Input: part model. Units: mm. Frame: model coordinates. A direction names the side the tool comes from. Give positions to 0.01 mm unless a question says otherwise; leave off trailing zeros. Loops run counter-clockwise (first coordinate to the right, second up) from the corner with the lowest first, then second, coordinate; pieces in that order, holes last. Notation, with made-up numbers: (72, 51) -> (78, 51) arc R24 cw to (78, 88) -> close; hole circle Ø11 at (29, 16.5). An arc over 180 degrees is marked (long way). One line per question, with ' | ' between items.
from build123d import *

# Parameters (mm, degrees)
SKETCH_1_R          = 1.45
EXTRUDE_1_DEPTH     = 1
SKETCH_2_W          = 3.674905937
SKETCH_2_H          = 8.103638732
EXTRUDE_2_DEPTH     = 4.6
SKETCH_3_W          = 9.2
SKETCH_3_H          = 9.2
EXTRUDE_3_DEPTH     = 3
SKETCH_4_R          = 3.75
EXTRUDE_4_DEPTH     = 3.8
SKETCH_5_W          = 5.32390219
SKETCH_5_H          = 6.666656283
EXTRUDE_5_DEPTH     = 2.2
SKETCH_6_W          = 12.46284852
SKETCH_6_H          = 12.975244807
EXTRUDE_6_DEPTH     = 1.7
SKETCH_7_W          = 10.69456342
SKETCH_7_H          = 13.354174441
EXTRUDE_7_DEPTH     = 1
SKETCH_8_W          = 14.555394544
SKETCH_8_H          = 14.555394544
EXTRUDE_8_DEPTH     = 6
SKETCH_9_W          = 18.172258066
SKETCH_9_H          = 5.460745639
EXTRUDE_9_DEPTH     = 2.5
SKETCH_10_W         = 17.57536677
SKETCH_10_H         = 2.2
CUT_EXTRUDE_1_DEPTH = 4.5


with BuildPart() as part:
    # 草图1 → 凸台-拉伸1 (new body)
    with BuildSketch(Plane(origin=(0, 0, 0), x_dir=(1, 0, 0), z_dir=(0, 1, 0))):
        with BuildLine():
            Line((-11, 17.5), (11, 17.5))
            ThreePointArc((11, 17.5), (11.707106781, 17.207106781), (12, 16.5))
            Line((12, 16.5), (12, 12.3))
            ThreePointArc((12, 12.3), (12.527207794, 11.027207794), (13.8, 10.5))
            Line((13.8, 10.5), (18, 10.5))
            ThreePointArc((18, 10.5), (18.707106781, 10.207106781), (19, 9.5))
            Line((19, 9.5), (19, -9.5))
            ThreePointArc((19, -9.5), (18.707106781, -10.207106781), (18, -10.5))
            Line((18, -10.5), (13.8, -10.5))
            ThreePointArc((13.8, -10.5), (12.527207794, -11.027207794), (12, -12.3))
            Line((12, -12.3), (12, -16.5))
            ThreePointArc((12, -16.5), (11.707106781, -17.207106781), (11, -17.5))
            Line((11, -17.5), (-11, -17.5))
            ThreePointArc((-11, -17.5), (-11.707106781, -17.207106781), (-12, -16.5))
            Line((-12, -16.5), (-12, -12.3))
            ThreePointArc((-12, -12.3), (-12.527207794, -11.027207794), (-13.8, -10.5))
            Line((-13.8, -10.5), (-18, -10.5))
            ThreePointArc((-18, -10.5), (-18.707106781, -10.207106781), (-19, -9.5))
            Line((-19, -9.5), (-19, 9.5))
            ThreePointArc((-19, 9.5), (-18.707106781, 10.207106781), (-18, 10.5))
            Line((-18, 10.5), (-13.8, 10.5))
            ThreePointArc((-13.8, 10.5), (-12.527207794, 11.027207794), (-12, 12.3))
            Line((-12, 12.3), (-12, 16.5))
            ThreePointArc((-12, 16.5), (-11.707106781, 17.207106781), (-11, 17.5))
        make_face()
        with Locations((15.875, 7.375)):
            Circle(SKETCH_1_R, mode=Mode.SUBTRACT)
        with Locations((15.875, -7.375)):
            Circle(SKETCH_1_R, mode=Mode.SUBTRACT)
        with Locations((-15.875, -7.375)):
            Circle(SKETCH_1_R, mode=Mode.SUBTRACT)
        with Locations((-15.875, 7.375)):
            Circle(SKETCH_1_R, mode=Mode.SUBTRACT)
    extrude(amount=EXTRUDE_1_DEPTH)

    # 草图2 → 凸台-拉伸2 (add)
    with BuildSketch(Plane(origin=(0, 1, 0), x_dir=(1, 0, 0), z_dir=(0, 1, 0))):
        with Locations((-17.008218503, 0.494698876)):
            Rectangle(SKETCH_2_W, SKETCH_2_H)
    extrude(amount=EXTRUDE_2_DEPTH)

    # 草图3 → 凸台-拉伸3 (add)
    with BuildSketch(Plane(origin=(0, 1, 0), x_dir=(1, 0, 0), z_dir=(0, 1, 0))):
        with Locations((0, 9.9)):
            Rectangle(SKETCH_3_W, SKETCH_3_H)
    extrude(amount=EXTRUDE_3_DEPTH)

    # 草图4 → 凸台-拉伸4 (add)
    with BuildSketch(Plane(origin=(0, 4, 0), x_dir=(1, 0, 0), z_dir=(0, 1, 0))):
        with Locations((0, 10.082434237)):
            Circle(SKETCH_4_R)
    extrude(amount=EXTRUDE_4_DEPTH)

    # 草图5 → 凸台-拉伸5 (add)
    with BuildSketch(Plane(origin=(0, 1, 0), x_dir=(1, 0, 0), z_dir=(0, 1, 0))):
        with Locations((16.560633805, 0.129563992)):
            Rectangle(SKETCH_5_W, SKETCH_5_H)
    extrude(amount=EXTRUDE_5_DEPTH)

    # 草图6 → 凸台-拉伸6 (add)
    with BuildSketch(Plane(origin=(0, 1, 0), x_dir=(1, 0, 0), z_dir=(0, 1, 0))):
        with Locations((0, -10.346273638)):
            Rectangle(SKETCH_6_W, SKETCH_6_H)
    extrude(amount=EXTRUDE_6_DEPTH)

    # 草图7 → 凸台-拉伸7 (add)
    with BuildSketch(Plane(origin=(0, 1, 0), x_dir=(1, 0, 0), z_dir=(0, 1, 0))):
        with Locations((0, -13.384558474)):
            Rectangle(SKETCH_7_W, SKETCH_7_H)
    extrude(amount=EXTRUDE_7_DEPTH)

    # 草图8 → 凸台-拉伸8 (add)
    with BuildSketch(Plane.XZ):
        Rectangle(SKETCH_8_W, SKETCH_8_H)
    extrude(amount=EXTRUDE_8_DEPTH)

    # 草图9 → 凸台-拉伸9 (add)
    with BuildSketch(Plane.XZ):
        with Locations((0, -13.73622766)):
            Rectangle(SKETCH_9_W, SKETCH_9_H)
    extrude(amount=EXTRUDE_9_DEPTH)

    # 草图10 → 切除-拉伸1 (cut)
    with BuildSketch(Plane.XZ.offset(6)):
        with Locations((-0.008749504, 5.958042987)):
            Rectangle(SKETCH_10_W, SKETCH_10_H)
        with Locations((-0.008749504, 2.958042987)):
            Rectangle(SKETCH_10_W, SKETCH_10_H)
        with Locations((-0.008749504, -0.041957013)):
            Rectangle(SKETCH_10_W, SKETCH_10_H)
        with Locations((-0.008749504, -3.041957013)):
            Rectangle(SKETCH_10_W, SKETCH_10_H)
        with Locations((-0.008749504, -6.041957013)):
            Rectangle(SKETCH_10_W, SKETCH_10_H)
    extrude(amount=-CUT_EXTRUDE_1_DEPTH, mode=Mode.SUBTRACT)


solid = part.part
1. Pin query (flat end, axial travel): P1, Ø4, axis at y = -3, z = 1.5, coming from the +X side; P2, Ø2.5, axis at y = 3, z = -10.5, coming from the +X side; P3, Ø1.7, axis at x = 15.875, z = 7.375, coming from the +Y side; P4, Ø1.8, axis at x = 3.5, y = -4, coming from the -Z side. Return the tip coordinate at first contact, or that it passes through.
Determined:
P1: stops at x = 7.28 | P2: stops at x = 4.6 | P3: passes through | P4: stops at z = -7.28
2. Section query B-B (x = 15.5). Output: boundary loops of the cut face in (y, z).
Determined:
outline: (0, -10.5) -> (1, -10.5) -> (1, -8.78) -> (0, -8.78) -> close; (0, -5.97) -> (1, -5.97) -> (1, -3.46) -> (3.2, -3.46) -> (3.2, 3.2) -> (1, 3.2) -> (1, 5.97) -> (0, 5.97) -> close; (0, 8.78) -> (1, 8.78) -> (1, 10.5) -> (0, 10.5) -> close
3. Section query C-C (x = -8). Output: boundary loops of the cut face in (y, z).
Determined:
outline: (-2.5, -16.47) -> (0, -16.47) -> (0, -17.5) -> (1, -17.5) -> (1, 17.5) -> (0, 17.5) -> (0, -11.01) -> (-2.5, -11.01) -> close
4. Ray query, line 1 along Y through (x, z) = (14, 9.5); line 2 along Y through (x, z) = (-6.5, -3.5); line 3 along X through (y, z) = (2, -7). Return the intervals inside material, ascending. Write a range as from..to.
Determined:
line 1: y = 0..1 | line 2: y = -1.5..1 | line 3: x = -4.6..4.6
5. Section query A-A (y = -5). Output: boundary loops of the cut face in (x, z), then the cut area to 3 significant figures.
Determined:
outline: (-7.28, -7.28) -> (7.28, -7.28) -> (7.28, -7.14) -> (-7.28, -7.14) -> close; (-7.28, -4.94) -> (7.28, -4.94) -> (7.28, -4.14) -> (-7.28, -4.14) -> close; (-7.28, -1.94) -> (7.28, -1.94) -> (7.28, -1.14) -> (-7.28, -1.14) -> close; (-7.28, 1.06) -> (7.28, 1.06) -> (7.28, 1.86) -> (-7.28, 1.86) -> close; (-7.28, 4.06) -> (7.28, 4.06) -> (7.28, 4.86) -> (-7.28, 4.86) -> close; (-7.28, 7.06) -> (7.28, 7.06) -> (7.28, 7.28) -> (-7.28, 7.28) -> close | area: 51.8 mm2
6. Reachability of faces 1 (the flat face through (0, 2, -5.3)), 2 (the flat face through (-17, 3, 3.557)), 3 (the flat face through (0, -4, 4.058)), 4 (the flat face through (9.086, -1, -14)) from +Z, -Z, +X, -X, +Y, -Y: full face, straight path, thin tool, end or side. Return the list, or none.
Determined:
face 1: +X, -X, +Y | face 2: +Z, +X, -X, +Y | face 3: +X, -X, -Y | face 4: +Z, -Z, +X, -Y
7. Pull-direction query (Z, two-part tool) for faces 5 (the flat face through (0, -4, -1.142)), 6 (the cylindrical face through (-0.81, 5.87, -6.42)), 7 (the cylindrical face through (-18.699, 0.493, 10.215)), 8 (the flat face through (0, 2, 18)); classes: pulls with the +Z half, pulls with the -Z half, needs draft (parallel to the pull), parting line crosses it, or undercut.
Determined:
face 5: undercut | face 6: parting line crosses it | face 7: pulls with the +Z half | face 8: needs draft
8. Section query D-D (x = 10.5). Output: boundary loops of the cut face in (y, z).
Determined:
outline: (0, -17.5) -> (1, -17.5) -> (1, 17.5) -> (0, 17.5) -> close
